Build history of the part. All positions in model axes, mm. Face numbers are marked on the shaded views. Give positions to 0.01 mm unless a question says otherwise; leave off trailing zeros. Order: outer loops, then holes, each group sorted by start corner. A loop starts at its lowest first (then second) coordinate and runs counter-clockwise, first axis right, second up. Notation, with made-up numbers: (66.25, 33) - (123.25, 33) arc R27 ccw to (123.25, 67) - close; hole circle Ø6 at (10.25, 59). An arc over 180 degrees is marked (long way). Write each question's results on one line, items separated by ' | '. Start each with the question number.
1) Cut at A-A on z = 0. List the corners of the cut face in (x, y), plus the area to 3 significant figures.
2) Drop flat-ended pins along their axis: pin 1 Ø6.5 at (y, z) = (0, 0) entering from -X; pin 2 Ø4 at (y, z) = (0.5, -2) entering from +X. Give the stop position or say it passes through.
3) Drill centre lines: line 1 along Y through (x, z) = (1.1, 0); line 2 along Z through (x, y) = (0.9, -3); line 3 along Y through (x, z) = (1.4, -1). Where is each one in solid material? Low to high. Write a range as from..to.
4) Two-plate mould, pull along Y, no slides. Class the marked faces 1, 2, 3 and 4: +Y half, -Y half, draft (parallel to the pull), parting line (faces both ways), or undercut.
5) Cut at B-B on x = 1. List the corners of the cut face in (y, z).
from build123d import *

# Parameters (mm, degrees)
EXTRUDE_1_DEPTH = 2.5


with BuildPart() as part:
    # Эскиз1 → Бобышка-Вытянуть1 (new body)
    with BuildSketch(Plane(origin=(0, 0, 0), x_dir=(0, 0, -1), z_dir=(1, 0, 0))):
        Polygon((6.350852961, 0), (3.175426481, 5.5), (-3.175426481, 5.5), (-6.350852961, 0), (-3.175426481, -5.5), (3.175426481, -5.5), align=None)
    extrude(amount=EXTRUDE_1_DEPTH)

    # Эскиз2 → Вырез-Повернуть1 (revolve, cut)
    with BuildSketch(Plane(origin=(0, 0, 0), x_dir=(1, 0, 0), z_dir=(0, 1, 0))):
        Polygon((0, 5.350852961), (0.267949192, 6.350852961), (2.232050808, 6.350852961), (2.5, 5.350852961), (4.577096119, 5.350852961), (4.577096119, 7.799096081), (-1.908033153, 7.799096081), (-1.908033153, 5.350852961), align=None)
    revolve(axis=Axis((0, 0, 0), (1, 0, 0)), mode=Mode.SUBTRACT)

    # Эскиз3 → Отверстие обработанное метчиком M8x1.01 (revolve, cut)
    with BuildSketch(Plane.ZX):
        Polygon((0, 0), (0, 2.5), (4.25, 2.5), (3.5, 1.974844346), (3.5, 0.525155654), (4.25, 0), align=None)
    revolve(axis=Axis((-6.35, 0, 0), (1, 0, 0)), mode=Mode.SUBTRACT)


solid = part.part
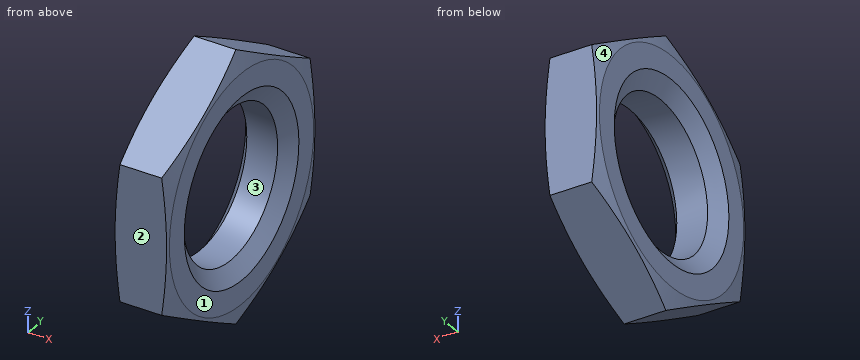
Results:
1) outline: (0, -5.35) - (0.04, -5.5) - (2.46, -5.5) - (2.5, -5.35) - (2.5, -4.25) - (1.97, -3.5) - (0.53, -3.5) - (0, -4.25) - close; (0, 4.25) - (0.53, 3.5) - (1.97, 3.5) - (2.5, 4.25) - (2.5, 5.35) - (2.46, 5.5) - (0.04, 5.5) - (0, 5.35) - close | area: 9.20 mm^2
2) pin 1: through | pin 2: x = 2.37
3) line 1: -5.5..-3.5, 3.5..5.5 | line 2: -4.62..-1.8, 1.8..4.62 | line 3: -5.5..-3.35, 3.35..5.5
4) face 1: draft | face 2: -Y half | face 3: undercut | face 4: parting line
5) outline: (-5.5, -3.18) - (0, -6.35) - (5.5, -3.18) - (5.5, 3.18) - (0, 6.35) - (-5.5, 3.18) - close; hole circle Ø7 at (0, 0)
